from build123d import *

# Parameters (mm, degrees)
F0_W     = 270
F0_H     = 42
F1_DEPTH = 6.35
F2_R     = 5
F3_DEPTH = 6.351
F4_R     = 3.3
F5_DEPTH = 6.351
F6_R     = 5.16
F7_DEPTH = 6.351
F8_R     = 1.25
F9_DEPTH = 6.351


with BuildPart() as f1:
    # F0 (on Top) → F1 (new body)
    with BuildSketch(Plane.XY):
        with Locations((135, 21)):
            Rectangle(F0_W, F0_H)
    extrude(amount=F1_DEPTH)

    # F2 (on face) → F3 (cut, through all)
    with BuildSketch(Plane.XY.offset(6.35)):
        with Locations((135, 21)):
            Circle(F2_R)
    extrude(amount=-F3_DEPTH, mode=Mode.SUBTRACT)

    # F4 (on face) → F5 (cut, through all)
    with BuildSketch(Plane.XY.offset(6.35)):
        with Locations((10, 21)):
            Circle(F4_R)
        with Locations((260, 21)):
            Circle(F4_R)
    extrude(amount=-F5_DEPTH, mode=Mode.SUBTRACT)

    # F6 (on face) → F7 (cut, through all)
    with BuildSketch(Plane.XY.offset(6.35)):
        with Locations((103.25, 21)):
            Circle(F6_R)
        with Locations((166.75, 21)):
            Circle(F6_R)
    extrude(amount=-F7_DEPTH, mode=Mode.SUBTRACT)

    # F8 (on face) → F9 (cut, through all)
    with BuildSketch(Plane.XY.offset(6.35)):
        with Locations((135, 29.32)):
            Circle(F8_R)
        with Locations((126.68, 21)):
            Circle(F8_R)
        with Locations((135, 12.68)):
            Circle(F8_R)
        with Locations((143.32, 21)):
            Circle(F8_R)
    extrude(amount=-F9_DEPTH, mode=Mode.SUBTRACT)


solid = f1.part
Geometry: final body of the model. Coordinates: model frame, mm. Round coordinates to 2 decimals unless told otherwise and drop trailing zeros. Write each loop counter-clockwise with the first axis right and the second up, starting at its lowest first coordinate (ties: lowest second). Pieces come first, ordered by that corner, then holes. Notation, with made-up numbers: M 41.25,33.25 L 100.25,33.25 A12 ccw 100.25,44.25 Z; hole C 77,-28 d4. An arc over 180 degrees is marked long. Write item = value, one per line.
Item 1: Section query A-A on x = 260. Return loops of the section in (y, z), then the cut area to 3 significant figures.
Findings:
outline = M 0,0 L 17.7,0 L 17.7,6.35 L 0,6.35 Z; M 24.3,0 L 42,0 L 42,6.35 L 24.3,6.35 Z
area = 225 mm^2
Item 2: Section query B-B on z = 1.75. State how many separate pieces and enclosed holes the cut face has, then the cut area to 3 significant figures.
Findings:
separate_pieces = 1
enclosed_holes = 9
area = 11,000 mm^2
Item 3: Material intervals for line 1 along Y through (x, z) = (135, 4.25); line 2 along Y through (x, z) = (166.5, 5.5); line 3 along X through (y, z) = (25, 3.75), sorted ascending. Write a range as [from, to].
Findings:
line_1 = [0, 11.43], [13.93, 16], [26, 28.07], [30.57, 42]
line_2 = [0, 15.85], [26.15, 42]
line_3 = [0, 99.99], [106.51, 132], [138, 163.49], [170.01, 270]
Item 4: Pull-direction query (Y, two-part tool) for faces 1 (the face through (133, 26, 0)), 2 (the face through (133, 0, 3)), 3 (the face through (137.307, 16.564, 3.219)); classes: pulls with the +Y half, pulls with the -Y half, needs draft (parallel to the pull), parting line crosses it, or undercut.
Findings:
face_1 = needs draft
face_2 = pulls with the -Y half
face_3 = undercut
Item 5: Pin query (flat end, axial travel): P1, Ø4, axis at x = 135, y = 12.68, coming from the +Z side; P2, Ø9, axis at x = 135, y = 21, coming from the +Z side. Return the tip coordinate at first contact, or that it passes through.
Findings:
P1 = 6.35
P2 = through
